from build123d import *

# Parameters (mm, degrees)
SKETCH1_R           = 25
BOSS_EXTRUDE1_DEPTH = 70
SKETCH2_OUTSIDE_W   = 71.9
SKETCH2_OUTSIDE_H   = 71.9
SKETCH2_OUTSIDE_R   = 13
CUT_EXTRUDE1_DEPTH  = 17
FILLET1_R           = 4


with BuildPart() as part:
    # Sketch1 → Boss-Extrude1 (new body)
    with BuildSketch(Plane(origin=(0, 0, 0), x_dir=(1, 0, 0), z_dir=(0, 1, 0))):
        with Locations(Location((0, 0, 0), (0, 0, 270))):
            Circle(SKETCH1_R)
    extrude(amount=BOSS_EXTRUDE1_DEPTH)

    # Sketch2 outside → Cut-Extrude1 (cut)
    with BuildSketch(Plane(origin=(0, 67, 0), x_dir=(1, 0, 0), z_dir=(0, 1, 0))):
        Rectangle(SKETCH2_OUTSIDE_W, SKETCH2_OUTSIDE_H)
        with Locations(Location((0, 0, 0), (0, 0, 270))):
            Circle(SKETCH2_OUTSIDE_R, mode=Mode.SUBTRACT)
    extrude(amount=-CUT_EXTRUDE1_DEPTH, mode=Mode.SUBTRACT)

    # Fillet1
    fillet1_edges = [part.edges().sort_by_distance(p)[0] for p in [
        (0, 67, -13),
        (0, 50, -13),
    ]]
    fillet(fillet1_edges, radius=FILLET1_R)


solid = part.part
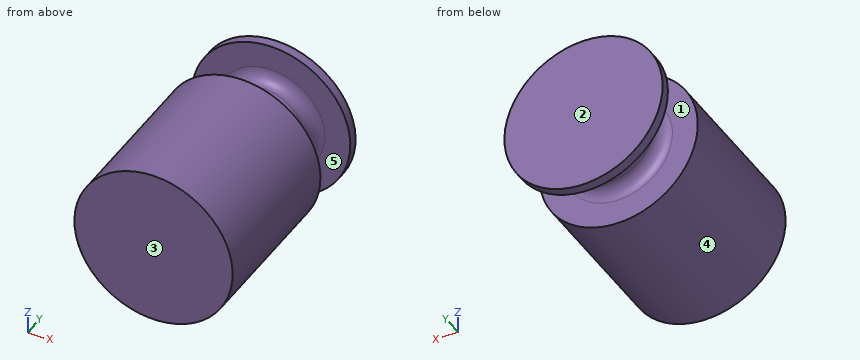
Design review of the part built by this model. Coordinates are the model's own, in mm. Face numbers are marked on the shaded views. A direction names the side the tool comes from. Give positions to 0.01 mm unless a question says otherwise; leave off trailing zeros. Write each loop counter-clockwise with the first axis right and the second up, starting at its lowest first coordinate (ties: lowest second). Pieces come first, ordered by that corner, then holes. Notation, with made-up numbers: M 62.25,10.5 L 106.25,10.5 A29 cw 106.25,33.5 Z; hole C 40,68 d7. An arc over 180 degrees is marked long. Return JSON: item names as keys, results as strings. Group by question number.
Item 1: The part is to be moulded in two halves that separate along Y. For the marked faces 1, 2 and 3, say which applies: pulls with the +Y half, pulls with the -Y half, needs draft (parallel to the pull), parting line crosses it, or undercut.
Item 2: Take a section at C-C (z = 0). Give the boundary of the cut face in (x, y).
Item 3: Take a section at B-B (x = -19). Give the boundary of the cut face in (y, z).
Item 4: Take a section at A-A (z = -21.5). Give the boundary of the cut face in (x, y).
Item 5: Tool access review of the marked faces 4 and 5: name each direction out of +Z, -Z, +X, -X, +Y, -Y from which nothing blocks a thin tool from reaching the whole face with its end or side.
Item 6: Take a section at D-D (y = 19). Give the boundary of the cut face in (x, z).
Item 7: Wall thickness on line 1 along Y through (x, z) = (17, 11); line 2 along Y through (x, z) = (-15, 2); line 3 along Z through (x, y) = (3.5, 31): over which ranges is each line inside the solid? List them lowest first.
Item 8: Clearance check with flat-ended pins moving along their axes: pin 1 Ø12 at (y, z) = (14, -8) entering from -X; pin 2 Ø5 at (x, y) = (-11.5, 31.5) entering from +Z; pin 3 Ø8 at (y, z) = (27.5, -11.5) entering from -X. State where each tip first meets the part, or that it passes through.
Return value:
{
 "1": {"face 1": "undercut", "face 2": "pulls with the +Y half", "face 3": "pulls with the -Y half"},
 "2": {"outline": "M -25,0 L 25,0 L 25,50 L 17,50 A4 cw 13,54 L 13,63 A4 cw 17,67 L 25,67 L 25,70 L -25,70 L -25,67 L -17,67 A4 cw -13,63 L -13,54 A4 cw -17,50 L -25,50 Z"},
 "3": {"outline": "M 0,-16.25 L 50,-16.25 L 50,16.25 L 0,16.25 Z; M 67,-16.25 L 70,-16.25 L 70,16.25 L 67,16.25 Z"},
 "4": {"outline": "M -12.76,0 L 12.76,0 L 12.76,50 L -12.76,50 Z; M -12.76,67 L 12.76,67 L 12.76,70 L -12.76,70 Z"},
 "5": {"face 4": "+Y, -Y", "face 5": "none"},
 "6": {"outline": "C 0,0 d50"},
 "7": {"line 1": "y = 0 to 50, 67 to 70", "line 2": "y = 0 to 50.46, 66.54 to 70", "line 3": "z = -24.75 to 24.75"},
 "8": {"pin 1": "stops at x = -24.92", "pin 2": "stops at z = 23.32", "pin 3": "stops at x = -23.85"}
}
